Verification items for the finished model (mm, model axes). Face numbers are marked on the shaded views. A direction names the side the tool comes from. Round coordinates to 2 decimals unless told otherwise and drop trailing zeros. Order: outer loops, then holes, each group sorted by start corner. A loop starts at its lowest first (then second) coordinate and runs counter-clockwise, first axis right, second up. Notation, with made-up numbers: M 44,34.25 L 84,34.25 A22 ccw 84,45.25 Z; hole C -13.75,87 d3. An arc over 180 degrees is marked long. Use one line per item in the form item = value. Start each with the question number.
Item 1: Release check for a two-part mould opening along X. For the marked faces 1, 2, 3 and 4 record: +X half, -X half, draft (parallel to the pull), parting line (faces both ways), or undercut.
Item 2: Thickness scan on probe 1 along X at (y, z) = (33.25, 10.5) (3 decimals); probe 2 along X at (y, z) = (17.5, 13); probe 3 along X at (y, z) = (2.5, 12.5). Record the ranges inside material, lowest first. Write a range as [from, to].
Item 3: Cross-section at C-C on y = 21. Enter the section's corners in (x, z), then the cut area to 3 significant figures.
Item 4: Cross-section at D-D on x = 17. Enter the section's corners in (y, z) (3 decimals).
Item 5: Go/stop test with flat-tipped pins: pin 1 Ø8 at (y, z) = (34.5, 0) entering from -X; pin 2 Ø3.5 at (y, z) = (1, -0.5) entering from -X; pin 3 Ø4 at (y, z) = (13, 0.5) entering from +X. Record where each tip stops, or that it passes through.
Item 6: Cross-section at B-B on x = 27.5. Enter the section's corners in (y, z) (3 decimals), then the cut area to 3 significant figures.
Item 7: Tool access check on the marked faces 5, 6, 7 and 8. Record the directions out of +Z, -Z, +X, -X, +Y, -Y that give a thin tool (end or side, any length) a straight path to the whole face; none if there is none.
Item 8: Cross-section at A-A on z = -7.5. Enter the section's corners in (x, y) (3 decimals).
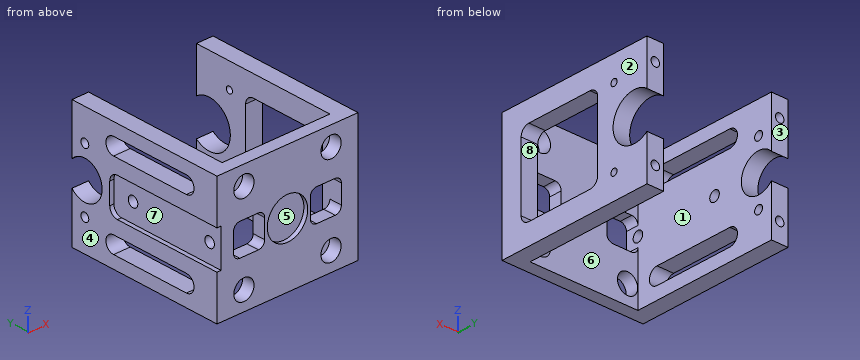
from build123d import *

# Parameters (mm, degrees)
EXTRUDE_1_DEPTH               = 15
CHAMFER_1_SIZE                = 10
SKETCH_2_R                    = 4.5
CUT_EXTRUDE_1_DEPTH           = 58.976288256
SKETCH_3_W                    = 20
SKETCH_3_H                    = 20
CUT_EXTRUDE_2_DEPTH           = 10
FILLET_1_R                    = 2
SKETCH_4_W                    = 9
SKETCH_4_H                    = 28
CUT_EXTRUDE_3_DEPTH           = 1
FILLET_2_R                    = 2
HOLE_WIZARD_M2_2_D            = 1.6
HOLE_WIZARD_M2_2_DEPTH        = 6
HOLE_WIZARD_M2_2_TIP          = 0.480688495
CUT_EXTRUDE_4_DEPTH           = 58.976288256
EXTRUDE_2_DEPTH               = 4
EXTRUDE_3_DEPTH               = 4
CUT_EXTRUDE_5_DEPTH           = 4
SKETCH_12_W                   = 7.5
SKETCH_12_H                   = 7.5
CUT_EXTRUDE_6_DEPTH           = 4
FILLET_3_R                    = 1.5
HOLE_WIZARD_M3_1_D            = 2.5
HOLE_WIZARD_M3_1_DEPTH        = 8.5
HOLE_WIZARD_M3_1_TIP          = 0.751075774
SKETCH_17_R                   = 4.875
CUT_EXTRUDE_8_DEPTH           = 1
FILLET_4_R                    = 1.5
HOLE_WIZARD_M2_5_1_AT_2_COUNT = 2
HOLE_WIZARD_M2_5_1_AT_2_PITCH = 21
HOLE_WIZARD_M2_5_2_D          = 2.05
HOLE_WIZARD_M2_5_2_DEPTH      = 6.25
HOLE_WIZARD_M2_5_2_TIP        = 0.615882135
SKETCH_24_R                   = 2.435
CUT_EXTRUDE_9_DEPTH           = 10
SKETCH_25_R                   = 5.5
CUT_EXTRUDE_10_DEPTH          = 10


with BuildPart() as part:
    # 草图1 → 凸台-拉伸1 (new, symmetric)
    with BuildSketch(Plane.XY):
        Polygon((0, 0), (34, 0), (34, 44.5), (30, 44.5), (30, 4), (30, 3), (4, 3), (4, 4), (4, 42), (0, 42), align=None)
    extrude(amount=EXTRUDE_1_DEPTH, both=True)

    # 倒角1
    chamfer_1_edges = [part.edges().sort_by_distance(p)[0] for p in [
        (32, 44.5, -15),
        (32, 44.5, 15),
        (2, 42, 15),
        (2, 42, -15),
    ]]
    chamfer(chamfer_1_edges, length=CHAMFER_1_SIZE)

    # 草图2 → 切除-拉伸1 (cut, through all)
    with BuildSketch(Plane(origin=(34, 0, 0), x_dir=(0, 0, -1), z_dir=(1, 0, 0))):
        with Locations((0, 34.5)):
            Circle(SKETCH_2_R)
    extrude(amount=-CUT_EXTRUDE_1_DEPTH, mode=Mode.SUBTRACT)

    # 草图3 → 切除-拉伸2 (cut)
    with BuildSketch(Plane(origin=(34, 0, 0), x_dir=(0, 0, -1), z_dir=(1, 0, 0))):
        with Locations((0, 15)):
            Rectangle(SKETCH_3_W, SKETCH_3_H)
    extrude(amount=-CUT_EXTRUDE_2_DEPTH, mode=Mode.SUBTRACT)

    # 圆角1
    fillet_1_edges = [part.edges().sort_by_distance(p)[0] for p in [
        (32, 25, -10),
        (32, 5, -10),
        (32, 5, 10),
        (32, 25, 10),
    ]]
    fillet(fillet_1_edges, radius=FILLET_1_R)

    # 草图4 → 切除-拉伸3 (cut)
    with BuildSketch(Plane.ZY):
        with Locations((0, 14)):
            Rectangle(SKETCH_4_W, SKETCH_4_H)
    extrude(amount=-CUT_EXTRUDE_3_DEPTH, mode=Mode.SUBTRACT)

    # 圆角2
    fillet_2_edges = [part.edges().sort_by_distance(p)[0] for p in [
        (0.5, 28, -4.5),
        (0.5, 28, 4.5),
    ]]
    fillet(fillet_2_edges, radius=FILLET_2_R)

    # M2 螺纹孔2
    with Locations(Plane(origin=(34, 29.25, 9.09326674), x_dir=(0, 0, 1), z_dir=(1, 0, 0))):
        with Locations((0, 0), (-18.18653348, 0)):
            Hole(HOLE_WIZARD_M2_2_D / 2, depth=HOLE_WIZARD_M2_2_DEPTH)
            with Locations((0, 0, -(HOLE_WIZARD_M2_2_DEPTH + HOLE_WIZARD_M2_2_TIP / 2))):  # 118° drill point
                Cone(0, HOLE_WIZARD_M2_2_D / 2, HOLE_WIZARD_M2_2_TIP, mode=Mode.SUBTRACT)

    # 草图5 → 切除-拉伸4 (cut, through all)
    with BuildSketch(Plane(origin=(34, 0, 0), x_dir=(0, 0, -1), z_dir=(1, 0, 0))):
        Polygon((-3, 37.854101966), (-15, 37.854101966), (-15, 44.5), (15, 44.5), (15, 37.854101966), align=None)
    extrude(amount=-CUT_EXTRUDE_4_DEPTH, mode=Mode.SUBTRACT)

    # 草图9 → 凸台-拉伸2 (add)
    with BuildSketch(Plane.ZY):
        Polygon((15, 32), (15, 37.854101966), (9.145898034, 37.854101966), align=None)
        Polygon((-15, 37.854101966), (-9.145898034, 37.854101966), (-15, 32), align=None)
    extrude(amount=-EXTRUDE_2_DEPTH)

    # 草图10 → 凸台-拉伸3 (add)
    with BuildSketch(Plane(origin=(34, 0, 0), x_dir=(0, 0, -1), z_dir=(1, 0, 0))):
        Polygon((11.645898034, 37.854101966), (15, 37.854101966), (15, 34.5), align=None)
        Polygon((-15, 34.5), (-15, 37.854101966), (-11.645898034, 37.854101966), align=None)
    extrude(amount=-EXTRUDE_3_DEPTH)

    # 草图11 → 切除-拉伸5 (cut)
    with BuildSketch(Plane.ZY):
        with BuildLine():
            Line((-8, 27), (-8, 8))
            ThreePointArc((-8, 8), (-10, 6), (-12, 8))
            Line((-12, 8), (-12, 27))
            ThreePointArc((-12, 27), (-10, 29), (-8, 27))
        make_face()
        with BuildLine():
            Line((8, 27), (8, 8))
            ThreePointArc((8, 8), (10, 6), (12, 8))
            Line((12, 8), (12, 27))
            ThreePointArc((12, 27), (10, 29), (8, 27))
        make_face()
    extrude(amount=-CUT_EXTRUDE_5_DEPTH, mode=Mode.SUBTRACT)

    # 草图12 → 切除-拉伸6 (cut)
    with BuildSketch(Plane.XZ):
        with Locations((7.75, 0)):
            Rectangle(SKETCH_12_W, SKETCH_12_H)
    cut_extrude_6 = extrude(amount=-CUT_EXTRUDE_6_DEPTH, mode=Mode.SUBTRACT)

    # 圆角3
    fillet_3_edges = [part.edges().sort_by_distance(p)[0] for p in [
        (11.5, 1.5, 3.75),
        (4, 1.5, -3.75),
        (11.5, 1.5, -3.75),
        (4, 1.5, 3.75),
    ]]
    fillet(fillet_3_edges, radius=FILLET_3_R)

    # M3 螺纹孔1
    with Locations(Plane(origin=(1, 23, 0), x_dir=(0, 0, -1), z_dir=(-1, 0, 0))):
        with Locations((0, 0), (0, 20)):
            Hole(HOLE_WIZARD_M3_1_D / 2, depth=HOLE_WIZARD_M3_1_DEPTH)
            with Locations((0, 0, -(HOLE_WIZARD_M3_1_DEPTH + HOLE_WIZARD_M3_1_TIP / 2))):  # 118° drill point
                Cone(0, HOLE_WIZARD_M3_1_D / 2, HOLE_WIZARD_M3_1_TIP, mode=Mode.SUBTRACT)

    # 草图17 → 切除-拉伸8 (cut)
    with BuildSketch(Plane.XZ):
        with Locations(Location((17, 0, 0), (0, 0, 270))):
            Circle(SKETCH_17_R)
    extrude(amount=-CUT_EXTRUDE_8_DEPTH, mode=Mode.SUBTRACT)

    # 镜向2: 切除-拉伸6 across plane
    add(cut_extrude_6.mirror(Plane.ZY.offset(-17)), mode=Mode.SUBTRACT)

    # 圆角4
    fillet_4_edges = [part.edges().sort_by_distance(p)[0] for p in [
        (22.5, 1.5, -3.75),
        (22.5, 1.5, 3.75),
        (30, 1.5, 3.75),
        (30, 1.5, -3.75),
    ]]
    fillet(fillet_4_edges, radius=FILLET_4_R)

    # 草图20 → M2.5 螺纹孔1 (revolve, cut)
    with BuildSketch(Plane(origin=(32, 37.854101966, 10.5), x_dir=(0, 0, 1), z_dir=(1, 0, 0))):
        Polygon((0, 0), (0, 6.865882135), (1.025, 6.25), (1.025, 0), align=None)
    hole_wizard_m2_5_1 = revolve(axis=Axis((32, 44.204101966, 10.5), (0, -1, 0)), mode=Mode.SUBTRACT)

    # M2.5 螺纹孔1 at 2: M2.5 螺纹孔1 ×2
    with Locations(*[(0, 0, -i * HOLE_WIZARD_M2_5_1_AT_2_PITCH) for i in range(1, HOLE_WIZARD_M2_5_1_AT_2_COUNT)]):
        add(hole_wizard_m2_5_1, mode=Mode.SUBTRACT)

    # 镜向3: M2.5 螺纹孔1 across plane
    add(hole_wizard_m2_5_1.mirror(Plane.ZY.offset(-17)), mode=Mode.SUBTRACT)

    # 镜向3 copy 1 sketch → 镜向3 copy 1 (revolve, cut)
    with BuildSketch(Plane(origin=(2, 37.854101966, -10.5), x_dir=(0, 0, 1), z_dir=(-1, 0, 0))):
        Polygon((0, 0), (0, -6.865882135), (1.025, -6.25), (1.025, 0), align=None)
    revolve(axis=Axis((2, 44.204101966, -10.5), (0, 1, 0)), mode=Mode.SUBTRACT)

    # M2.5 螺纹孔2
    with Locations(Plane(origin=(0, 34.5, 7.5), x_dir=(0, 0, -1), z_dir=(-1, 0, 0))):
        with Locations((0, 0), (15, 0)):
            Hole(HOLE_WIZARD_M2_5_2_D / 2, depth=HOLE_WIZARD_M2_5_2_DEPTH)
            with Locations((0, 0, -(HOLE_WIZARD_M2_5_2_DEPTH + HOLE_WIZARD_M2_5_2_TIP / 2))):  # 118° drill point
                Cone(0, HOLE_WIZARD_M2_5_2_D / 2, HOLE_WIZARD_M2_5_2_TIP, mode=Mode.SUBTRACT)

    # 草图24 → 切除-拉伸9 (cut)
    with BuildSketch(Plane.XZ):
        with Locations(Location((6.5, 10.5, 0), (0, 0, 270))):
            Circle(SKETCH_24_R)
        with Locations(Location((27.5, 10.5, 0), (0, 0, 270))):
            Circle(SKETCH_24_R)
        with Locations(Location((6.5, -10.5, 0), (0, 0, 270))):
            Circle(SKETCH_24_R)
        with Locations(Location((27.5, -10.5, 0), (0, 0, 270))):
            Circle(SKETCH_24_R)
    extrude(amount=-CUT_EXTRUDE_9_DEPTH, mode=Mode.SUBTRACT)

    # 草图25 → 切除-拉伸10 (cut)
    with BuildSketch(Plane(origin=(34, 0, 0), x_dir=(0, 0, -1), z_dir=(1, 0, 0))):
        with Locations((0, 34.5)):
            Circle(SKETCH_25_R)
    extrude(amount=-CUT_EXTRUDE_10_DEPTH, mode=Mode.SUBTRACT)


solid = part.part
Output values:
q1.face_1 = undercut
q1.face_2 = +X half
q1.face_3 = draft
q1.face_4 = -X half
q2.probe_1 = [0, 0.975], [3.025, 4], [30, 30.975], [33.025, 34]
q2.probe_2 = [0, 4], [30, 34]
q2.probe_3 = [0, 5.11], [7.89, 26.11], [28.89, 34]
q3.outline = M 0,-15 L 4,-15 L 4,-12 L 0,-12 Z; M 0,-8 L 4,-8 L 4,8 L 0,8 L 0,4.5 L 1,4.5 L 1,-4.5 L 0,-4.5 Z; M 0,12 L 4,12 L 4,15 L 0,15 Z; M 30,-15 L 34,-15 L 34,-10 L 30,-10 Z; M 30,10 L 34,10 L 34,15 L 30,15 Z
q3.area = 119 mm2
q4.outline = M 0,-15 L 3,-15 L 3,15 L 0,15 L 0,4.875 L 1,4.875 L 1,-4.875 L 0,-4.875 Z
q5.pin_1 = through
q5.pin_2 = 1
q5.pin_3 = 4
q6.outline = M 0,-15 L 3,-15 L 3,-12.935 L 0,-12.935 Z; M 0,-8.065 L 3,-8.065 L 3,-3.75 L 0,-3.75 Z; M 0,3.75 L 3,3.75 L 3,8.065 L 0,8.065 Z; M 0,12.935 L 3,12.935 L 3,15 L 0,15 Z
q6.area = 38.3 mm2
q7.face_5 = -Y
q7.face_6 = +Z, -Z, +Y
q7.face_7 = -X, -Y
q7.face_8 = +X
q8.outline = M 0,0 L 34,0 L 34,5 L 30,5 L 30,3 L 4,3 L 4,33.475 L 0,33.475 Z; M 0,35.525 L 4,35.525 L 4,37.854 L 0,37.854 Z; M 30,25 L 34,25 L 34,37.854 L 30,37.854 Z
